The model under review builds one solid part; all positions refer to its coordinate system, in mm. A direction names the side the tool comes from. Coordinates: 2 decimals unless noted, no trailing zeros. Write each loop counter-clockwise with the first axis right and the second up, starting at its lowest first coordinate (ties: lowest second). Pieces come first, ordered by that corner, then holes. Notation, with made-up numbers: M 58.25,62 L 101.25,62 A32 cw 101.25,89 Z; hole C 4.5,-10 d4. An arc over 180 degrees is marked long. Answer as a JSON object with one key per item and string values.
```python
from build123d import *

# Parameters (mm, degrees)
SKETCH_1_R          = 16
EXTRUDE_1_DEPTH     = 2
SKETCH_2_R          = 13.945
EXTRUDE_2_DEPTH     = 11
SKETCH_3_R          = 16
EXTRUDE_3_DEPTH     = 2
SKETCH_4_R          = 5
CUT_EXTRUDE_1_DEPTH = 15
SKETCH_5_R          = 2
CUT_EXTRUDE_2_DEPTH = 20
SKETCH_8_R          = 2
CUT_EXTRUDE_3_DEPTH = 20


with BuildPart() as part:
    # 草图1 → 凸台-拉伸1 (new body)
    with BuildSketch(Plane.XY):
        Circle(SKETCH_1_R)
    extrude(amount=EXTRUDE_1_DEPTH)

    # 草图2 → 凸台-拉伸2 (add)
    with BuildSketch(Plane.XY.offset(2)):
        Circle(SKETCH_2_R)
    extrude(amount=EXTRUDE_2_DEPTH)

    # 草图3 → 凸台-拉伸3 (add)
    with BuildSketch(Plane.XY.offset(13)):
        Circle(SKETCH_3_R)
    extrude(amount=EXTRUDE_3_DEPTH)

    # 草图4 → 切除-拉伸1 (cut)
    with BuildSketch(Plane.XY.offset(15)):
        Circle(SKETCH_4_R)
    extrude(amount=-CUT_EXTRUDE_1_DEPTH, mode=Mode.SUBTRACT)

    # 草图5 → 切除-拉伸2 (cut)
    with BuildSketch(Plane(origin=(0, 0, 0), x_dir=(1, 0, 0), z_dir=(0, 1, 0))):
        with Locations(Location((0, -7.5, 0), (0, 0, 270))):
            Circle(SKETCH_5_R)
    extrude(amount=-CUT_EXTRUDE_2_DEPTH, mode=Mode.SUBTRACT)

    # 草图8 → 切除-拉伸3 (cut)
    with BuildSketch(Plane(origin=(0, 0, 0), x_dir=(0, 0, -1), z_dir=(1, 0, 0))):
        with Locations((-7.5, 0)):
            Circle(SKETCH_8_R)
    extrude(amount=-CUT_EXTRUDE_3_DEPTH, mode=Mode.SUBTRACT)


solid = part.part
```
(1) Add section A-A on x = 0. Give the boundary of the cut face in (y, z) (3 decimals), and give its area (3 significant figures).
Results list:
{"outline": "M -16,0 L -5,0 L -5,5.5 L -13.945,5.5 L -13.945,2 L -16,2 Z; M -16,13 L -13.945,13 L -13.945,9.5 L -5,9.5 L -5,15 L -16,15 Z; M 5,0 L 16,0 L 16,2 L 13.945,2 L 13.945,13 L 16,13 L 16,15 L 5,15 Z", "area": "249 mm²"}
(2) Draft analysis for pull direction X (two halves, no side actions). For faces 4 (the face through (-3.47, -15.62, 13.99)), 5 (the face through (1.1, 14.3, 13)), 6 (the face through (0.088, -9.2, 5.502)), state which applies: released by +X, released by -X, zero draft, split by the parting line, or undercut.
Results list:
{"face 4": "split by the parting line", "face 5": "zero draft", "face 6": "undercut"}
(3) Add section C-C on z = 7. Give the boundary of the cut face in (x, y) (1 decimal), and give its area (3 significant figures).
Results list:
{"outline": "M -13.8,-1.9 A13.9 ccw -1.9,-13.8 L -1.9,-4.6 A5 cw -4.6,-1.9 Z; M -13.8,1.9 L -4.6,1.9 A5 cw long 1.9,-4.6 L 1.9,-13.8 A13.9 ccw long Z", "area": "462 mm²"}
(4) For pin 1 Ø6.5 at (y, z) = (0, 7.5) entering from +X (3 decimals); pin 2 Ø3 at (x, y) = (-3.5, 0.5) entering from -Z; pin 3 Ø5 at (x, z) = (0, 7.5) entering from +Y (3 decimals); pin 4 Ø5 at (y, z) = (-8.5, 7) entering from -X, all flat-tipped, find the tip position at first contact; note any pin that passes through.
Results list:
{"pin 1": "x = 13.945", "pin 2": "z = 0", "pin 3": "y = 13.945", "pin 4": "x = -12.59"}
(5) For faces 1 (the face through (13.3, 4.19, 7.42)), 2 (the face through (-3.47, -15.62, 0.99)), 3 (the face through (-9.198, 0.088, 9.498)), list the 3-axis set-ups (+Z, -Z, +X, -X, +Y, -Y) from which the entire face can be reached by the end or side of a thin tool; tool diameter is ignored.
Results list:
{"face 1": "none", "face 2": "+Z, -Z", "face 3": "-X"}
(6) Wall thickness on line 1 along Z through (x, y) = (0, -8); line 2 along Y through (x, z) = (0, 11.25) (3 decimals); line 3 along Z through (x, y) = (14, 1): over which ranges is each line inside the solid? List them lowest first. Write a range as from..to.
Results list:
{"line 1": "0..5.5, 9.5..15", "line 2": "-13.945..-5, 5..13.945", "line 3": "0..2, 13..15"}
(7) Add section D-D on x = -8.5. Give the boundary of the cut face in (y, z) (3 decimals).
Results list:
{"outline": "M -13.555,0 L 13.555,0 L 13.555,2 L 11.055,2 L 11.055,13 L 13.555,13 L 13.555,15 L -13.555,15 L -13.555,13 L -11.055,13 L -11.055,2 L -13.555,2 Z; hole C 0,7.5 d4"}
